Part model, mm, in its own coordinate system. A direction names the side the tool comes from. Coordinates: 2 decimals unless noted, no trailing zeros. Order: outer loops, then holes, each group sorted by start corner. A loop starts at its lowest first (then second) coordinate and runs counter-clockwise, first axis right, second up.
```python
from build123d import *

# Parameters (mm, degrees)
SKETCH1_R           = 1.5
BOSS_EXTRUDE1_DEPTH = 3
EXTRUDE_1_DEPTH     = 3
EXTRUDE_2_DEPTH     = 3
EXTRUDE_3_REACH     = 100.745


with BuildPart() as part:
    # Sketch1 → Boss-Extrude1 (new body)
    # profile 1 of 2: a face of its own
    with BuildSketch(Plane.XY):
        with BuildLine():
            Line((20.05, 5), (0, 5))
            ThreePointArc((0, 5), (-5, 0), (0, -5))
            Line((0, -5), (22, -5))
            Line((22, -5), (25.516973514, -3.553997369))
            ThreePointArc((25.516973514, -3.553997369), (26.624391141, 1.901317064), (22, 5))
            Line((22, 5), (20.05, 5))
        make_face()
        Circle(SKETCH1_R, mode=Mode.SUBTRACT)
        with Locations((22, 0)):
            Circle(SKETCH1_R, mode=Mode.SUBTRACT)
    # profile 2 of 2: a face of its own
    with BuildSketch(Plane.XY):
        with BuildLine():
            Line((46.409029503, 15.837507263), (20.05, 5))
            Line((20.05, 5), (22, 5))
            ThreePointArc((22, 5), (26.624391141, 1.901317064), (25.516973514, -3.553997369))
            Line((25.516973514, -3.553997369), (48.359029503, 5.837507263))
            Line((48.359029503, 5.837507263), (58.872830999, 10.16025367))
            Line((58.872830999, 10.16025367), (53.359871826, 12.67140304))
            Line((53.359871826, 12.67140304), (46.409029503, 15.837507263))
        make_face()
    extrude(amount=BOSS_EXTRUDE1_DEPTH)

    # 草图1 → 凸台-拉伸1 (add)
    with BuildSketch(Plane.XY.offset(3)):
        Polygon((46.409029503, 15.837507263), (58.872830999, 10.16025367), (111.008388469, 31.59577286), (98.544586973, 37.273026453), align=None)
    extrude(amount=-EXTRUDE_1_DEPTH)

    # 草图4 → 凸台-拉伸2 (add)
    with BuildSketch(Plane(origin=(0, 0, 0), x_dir=(-1, 0, 0), z_dir=(0, 0, -1))):
        with BuildLine():
            Line((-111.008388469, 31.59577286), (-98.544586973, 37.273026453))
            Line((-98.544586973, 37.273026453), (-19.990187018, 4.97540791))
            Line((-19.990187018, 4.97540791), (-21.063636635, 2.318021494))
            ThreePointArc((-21.063636635, 2.318021494), (-24.318021494, 0.936363365), (-22.936363365, -2.318021494))
            Line((-22.936363365, -2.318021494), (-23.732077199, -4.287856967))
            Line((-23.732077199, -4.287856967), (-111.008388469, 31.59577286))
        make_face()
    extrude(amount=EXTRUDE_2_DEPTH)

    # 凸台-拉伸3: up to this plane
    extrude_3_end = Plane(origin=(98.544586973, 37.273026453, -70.058401543), z_dir=(0.4145222599320868, 0.9100391727946636, 0))
    # 草图5 → 凸台-拉伸3 (add, up to the surface)
    with BuildSketch(Plane(origin=(18.913747244, 7.640196631, 0), x_dir=(0.3745453459539944, -0.9272085977945863, 0), z_dir=(-0.9272085977945863, -0.3745453459539944, 0)), mode=Mode.PRIVATE) as extrude_3_sk1:
        with BuildLine():
            Line((17.949999281, -3), (17.949999281, -4))
            ThreePointArc((17.949999281, -4), (-0.050000719, -22), (17.949999281, -40))
            Line((17.949999281, -40), (17.949999281, -41))
            ThreePointArc((17.949999281, -41), (0.910251194, -30.405176091), (2.873990521, -10.43652475))
            Line((2.873990521, -10.43652475), (2.873990521, -3))
            Line((2.873990521, -3), (17.949999281, -3))
        make_face()
    extrude_3_tool1 = split(extrude(extrude_3_sk1.sketch, amount=-EXTRUDE_3_REACH, mode=Mode.PRIVATE), bisect_by=extrude_3_end, keep=Keep.BOTH, mode=Mode.PRIVATE)
    add(extrude_3_tool1.solids().sort_by_distance((20.149314, 4.581481, -6.718262))[0])


solid = part.part
```
(1) Drop flat-ended pins along their axis: pin 1 (10 mm diameter, centred on x = 25, z = -10.5, fed in from -Y); pin 2 (3.5 mm diameter, centred on x = 22, y = 0, fed in from +Z); pin 3 (3.5 mm diameter, centred on x = 6.5, z = 2, fed in from -Y); pin 4 (6 mm diameter, centred on y = 34, z = -36, fed in from +X). Give the stop position or say it passes through.
(2) Probe line 1 (Y direction, x = 0, z = 1); line 2 (Y direction, x = 22, z = 1); line 3 (Z direction, x = 107.5, y = 32). List the from-to ranges inside material, lowest first.
(3) Slice it at C-C, the plane z = -21.5. Give the cut face in (x, y), then the cut area to 3 significant figures.
(4) Pull direction Z, two halves, no side cores. Call faces 1 (the face through (20.5, 0.07, 1.48)), 2 (the face through (53, 13, 3)), 3 (the face through (23, 0, -3)): +Z half, -Z half, draft (parallel to the pull), parting line (faces both ways), or undercut.
(5) Slice it at A-A, the plane y = 0. State how many separate pieces and enclosed holes the cut face has, then the cut area to 3 significant figures.
(6) Tool access for faces 4 (the face through (10, 5, 1)), 5 (the face through (70, 12, -3)), 6 (the face through (59.82, 21.35, 0.04)), 7 (the face through (59.04, 20.75, -6.77)): list every direction of +Z, -Z, +X, -X, +Y, -Y with a clear straight run to the whole face (end or side of a thin tool).
(7) Slice it at B-B, the plane z = -30. Give the cut face in (x, y), then the cut area to 3 significant figures.
Here are the results:
1. pin 1: stops at y = -1.67
1. pin 2: stops at z = 3
1. pin 3: stops at y = -5
1. pin 4: stops at x = 109.22
2. line 1: y = -5 to -1.5, 1.5 to 5
2. line 2: y = -5 to -1.5, 1.5 to 5.8
2. line 3: z = -39.52 to -38.43, -5.57 to 3
3. outline: (18.52, 8.61) - (18.9, 7.68) - (95.54, 38.64) - (94.29, 39.21) - close
3. area: 82.2 mm2
4. face 1: draft
4. face 2: +Z half
4. face 3: undercut
5. separate pieces: 4
5. enclosed holes: 0
5. area: 205 mm2
6. face 4: +Z, -Z, -X, +Y
6. face 5: +Z, +X, -Y
6. face 6: +Z, -X, +Y
6. face 7: -X, +Y
7. outline: (19.18, 6.98) - (19.6, 5.95) - (97.89, 37.57) - (96.5, 38.21) - close
7. area: 93.1 mm2
